Drawing for the job (mm, zero at the part's lowest x, y, z). A direction names the side the tool comes from. Give positions to 0.01 mm unless a question says otherwise; leave off trailing zeros. Loops run counter-clockwise (first coordinate to the right, second up) from the corner with the lowest first, then second, coordinate; pieces in that order, holes last. Notation, with made-up numbers: (60.5, 19) -> (99.5, 19) arc R10 ccw to (99.5, 33) -> close; hole circle Ø10 at (39, 42). An arc over 180 degrees is marked (long way). Answer in a Markdown table with one row per item. Add a question column.
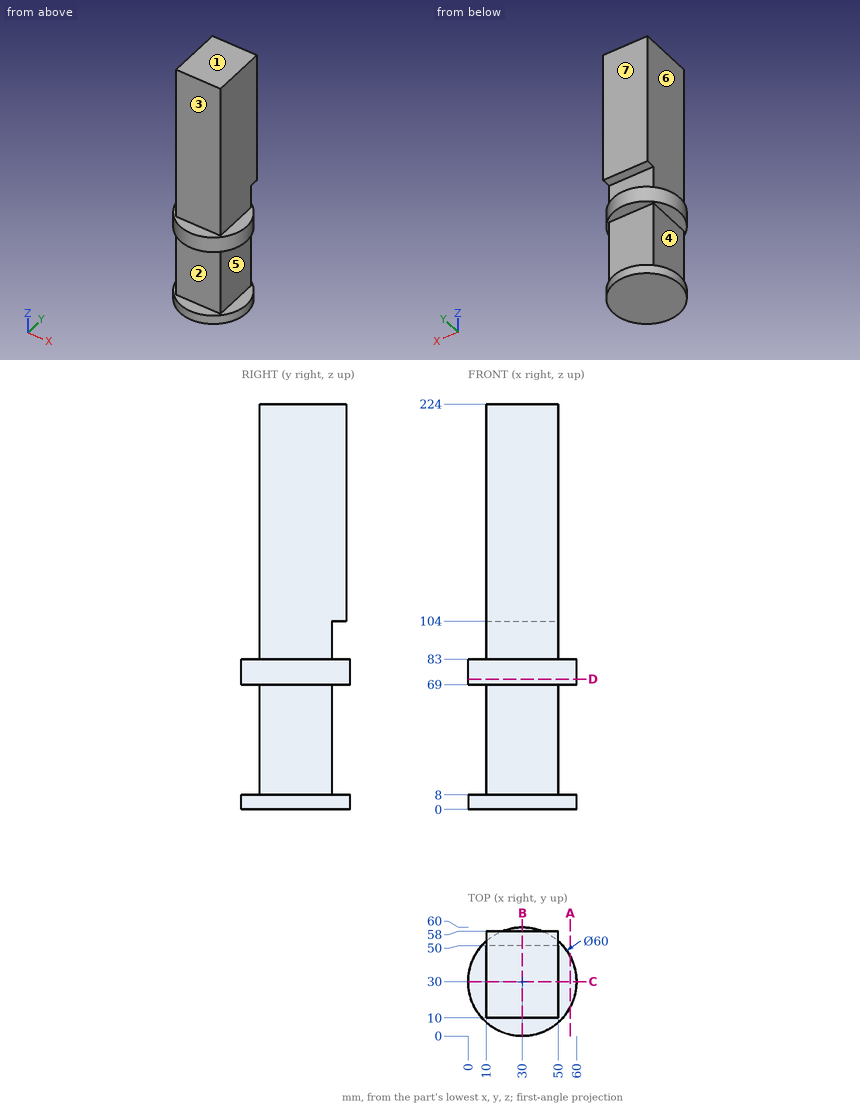
(1) Saw through at D-D, the plane z = 72. List the corners of the cut face in (x, y).
(2) Wall check: line 1 along Z through (x, y) = (55, 32); line 2 along X through (y, z) = (33.5, 96.5); line 3 along Y through (x, z) = (13, 156). Give the ranges that are in metal, low to high. Write a range as from..to.
(3) Flat gauge pins, fed straight in: pin 1 Ø6 at (x, z) = (46, 23) entering from -Y; pin 2 Ø6.5 at (x, z) = (26, 98.5) entering from +Y; pin 3 Ø4 at (x, z) = (40.5, 69) entering from +Y. Where does each tip first touch, or does it go through?
(4) Two-plate mould, pull along Z, no slides. Class the marked faces 1, 2 and 3: released by +Z, released by -Z, zero draft, split by the parting line, or undercut.
(5) Saw through at C-C, the plane y = 30. List the corners of the cut face in (x, z).
(6) 3-axis set-ups, long thin cutter, end or side, ignore diameter. For the marked faces 4, 5, 6 and 7: which of +Z, -Z, +X, -X, +Y, -Y reach the whole face in a straight line?
(7) Saw through at B-B, the plane x = 30. List the corners of the cut face in (y, z), then the cut area to 3 significant figures.
(8) Saw through at A-A, the plane x = 56.5. List the corners of the cut face in (y, z), then the cut area to 3 significant figures.
Worked answers:
| question | item | result |
|---|---|---|
| 1 | outline | circle Ø60 at (30, 30) |
| 2 | line 1 | 0..8, 69..83 |
| 2 | line 2 | 10..50 |
| 2 | line 3 | 10..58 |
| 3 | pin 1 | y = 10 |
| 3 | pin 2 | y = 50 |
| 3 | pin 3 | y = 58.77 |
| 4 | face 1 | released by +Z |
| 4 | face 2 | undercut |
| 4 | face 3 | zero draft |
| 5 | outline | (0, 0) -> (60, 0) -> (60, 8) -> (50, 8) -> (50, 69) -> (60, 69) -> (60, 83) -> (50, 83) -> (50, 224) -> (10, 224) -> (10, 83) -> (0, 83) -> (0, 69) -> (10, 69) -> (10, 8) -> (0, 8) -> close |
| 6 | face 4 | -X, +Y, -Y |
| 6 | face 5 | +X, +Y, -Y |
| 6 | face 6 | +Z, -X, +Y, -Y |
| 6 | face 7 | +Z, +X, -X, +Y |
| 7 | outline | (0, 0) -> (60, 0) -> (60, 8) -> (50, 8) -> (50, 69) -> (60, 69) -> (60, 83) -> (50, 83) -> (50, 104) -> (58, 104) -> (58, 224) -> (10, 224) -> (10, 83) -> (0, 83) -> (0, 69) -> (10, 69) -> (10, 8) -> (0, 8) -> close |
| 7 | area | 10,400 mm^2 |
| 8 | outline | (15.94, 0) -> (44.06, 0) -> (44.06, 8) -> (15.94, 8) -> close; (15.94, 69) -> (44.06, 69) -> (44.06, 83) -> (15.94, 83) -> close |
| 8 | area | 619 mm^2 |
